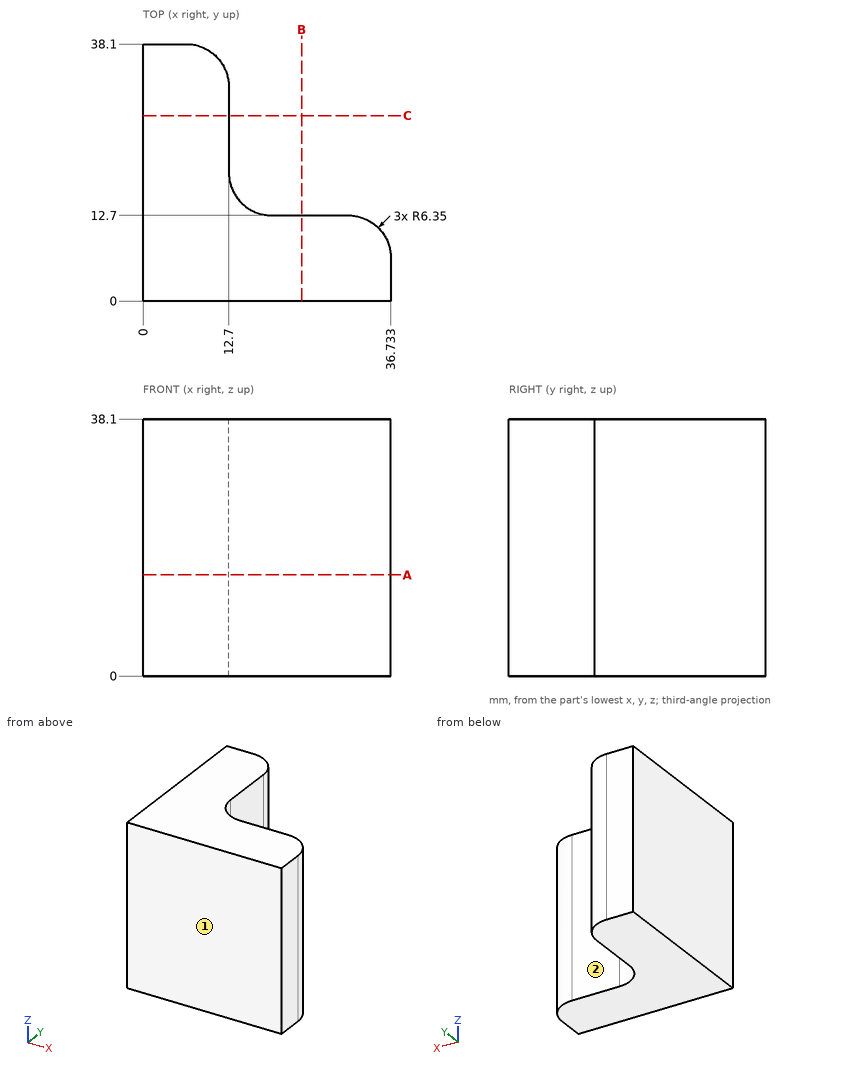
Verification items for this drawing (mm, ordinates from the low corner). A direction names the side the tool comes from. Round coordinates to 2 decimals unless told otherwise and drop trailing zeros. Order: outer loops, then holes, each group sorted by start corner. A loop starts at its lowest first (then second) coordinate and runs counter-clockwise, first axis right, second up. Notation, with made-up numbers: (51.5, -7.5) - (89.5, -7.5) arc R22 cw to (89.5, 3.5) - close; hole circle Ø7 at (-33, 32.25). An arc over 180 degrees is marked (long way). Answer as CSV lines item,"result". Start each with the question number.
1) Scan lines: probe 1 along Y at (x, z) = (6.5, 4); probe 2 along X at (y, z) = (32, 9) (1 decimal). Record each from-to range of solid material in increasing order.
2) Tool access check on the marked faces 1 and 2. Record the directions out of +Z, -Z, +X, -X, +Y, -Y that give a thin tool (end or side, any length) a straight path to the whole face; none if there is none.
3) Depth check by flat-ended pin: pin 1 (9 mm diameter, centred on x = 23.5, z = 28, fed in from +Y); pin 2 (1 mm diameter, centred on y = 25.5, z = 12.5, fed in from +X); pin 3 (12 mm diameter, centred on y = 24, z = 29, fed in from +X). Enter the tip coordinate at first touch or a pass-through.
4) Section check A-A (z = 15). Record the cut outline in (x, y).
5) Section check B-B (x = 23.5). Record the cut outline in (y, z).
Determined:
1,probe 1,"0 to 38.1"
1,probe 2,"0 to 12.7"
2,face 1,"+Z, -Z, +X, -X, -Y"
2,face 2,"+Z, -Z, +X, +Y"
3,pin 1,"y = 12.7"
3,pin 2,"x = 12.7"
3,pin 3,"x = 12.79"
4,outline,"(0, 0) - (36.73, 0) - (36.73, 6.35) arc R6.35 ccw to (30.38, 12.7) - (19.05, 12.7) arc R6.35 cw to (12.7, 19.05) - (12.7, 31.75) arc R6.35 ccw to (6.35, 38.1) - (0, 38.1) - close"
5,outline,"(0, 0) - (12.7, 0) - (12.7, 38.1) - (0, 38.1) - close"
